Design review of the part built by this model. Coordinates are the model's own, in mm. Face numbers are marked on the shaded views. Give positions to 0.01 mm unless a question says otherwise; leave off trailing zeros. Order: outer loops, then holes, each group sorted by start corner. A loop starts at its lowest first (then second) coordinate and runs counter-clockwise, first axis right, second up. Notation, with made-up numbers: (87.25, -21) -> (98.25, -21) arc R23 cw to (98.25, -13) -> close; hole circle Ø4 at (-22, 84.5). An arc over 180 degrees is marked (long way). One line per item, written item: value.
Autodesk Inventor part; units mm, degrees
ref_plane "YZ Plane" through (0, 0, 0) normal (1, 0, 0) x (0, 1, 0)
ref_plane "XZ Plane" through (0, 0, 0) normal (0, 1, 0) x (-1, 0, 0)
ref_plane "XY Plane" through (0, 0, 0) normal (0, 0, 1) x (1, 0, 0)
sketch "Sketch1" plane through (0, 0, 0) normal (1, 0, 0) x (0, 1, 0)
  line L0 (0, 0) -> (10, 0)
  line L1 (10, 0) -> (10, -3.5)
  line L2 (10, -3.5) -> (0, -3.5)
  line L3 (0, -3.5) -> (0, 0)
  line L4 (10, -3.5) -> (0, -3.5)
  line L5 (0, -3.5) -> (0, -6)
  line L6 (0, -6) -> (10, -6)
  line L7 (10, -6) -> (10, -3.5)
  line L8 (10, -6) -> (0, -6)
  line L9 (0, -6) -> (0, -9.5)
  line L10 (0, -9.5) -> (10, -9.5)
  line L11 (10, -9.5) -> (10, -6)
  line L12 (10, -9.5) -> (0, -9.5)
  line L13 (0, -9.5) -> (0, -12)
  line L14 (0, -12) -> (10, -12)
  line L15 (10, -12) -> (10, -9.5)
  line L16 (10, -12) -> (0, -12)
  line L17 (0, -12) -> (0, -15.5)
  line L18 (0, -15.5) -> (10, -15.5)
  line L19 (10, -15.5) -> (10, -12)
  line L20 (10, -7.75) -> (5, -7.75)
  circle A0 centre (5, -7.75) radius 1.75
  line L21 (6.75, -9.5) -> (3.25, -9.5)
  line L22 (3.25, -9.5) -> (3.25, -6)
  line L23 (3.25, -6) -> (6.75, -6)
  line L24 (6.75, -6) -> (6.75, -9.5)
  line L25 (6.75, -9.5) -> (3.25, -6) construction
  line L26 (3.25, -9.5) -> (6.75, -6) construction
  dimension "d0" = 10
  dimension "d1" = 3.5
  dimension "d2" = 2.5
  dimension "d3" = 3.5
  dimension "d4" = 2.5
  dimension "d5" = 3.5
  dimension "d8" = 3.5
  dimension "d11" = 3.5
extrude "Extrusion1" add sketch "Sketch1" along normal blind 2 contours L0 L1 L2 L3 | L2 L7 L6 L5 | L6 L22 L10 L9 | L11 L20 L24 L6 | L6 A0 L22 | L10 L15 L14 L13 | L24 A0 L6 | L11 L10 L24 L20 | A0 L10 L22 | L14 L19 L18 L17 | L24 L10 A0
properties part number "yellow_plate_screw_grip_2"
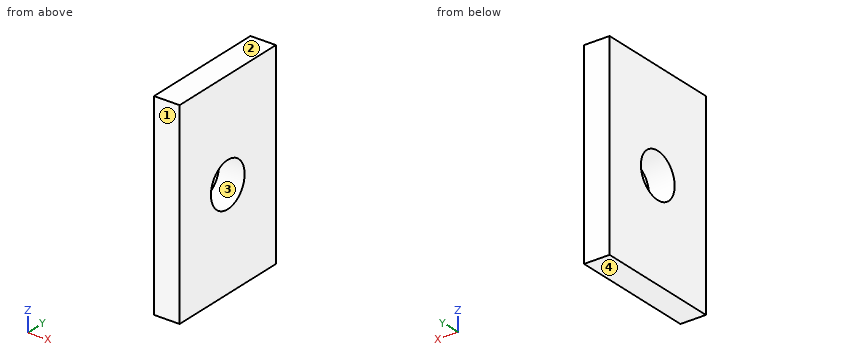
Item 1: Add section A-A on z = -7.75. Give the boundary of the cut face in (x, y).
Returned:
outline: (0, 0) -> (2, 0) -> (2, 3.25) -> (0, 3.25) -> close; (0, 6.75) -> (2, 6.75) -> (2, 10) -> (0, 10) -> close
Item 2: Add section B-B on y = 5. Give the boundary of the cut face in (x, z).
Returned:
outline: (0, -15.5) -> (2, -15.5) -> (2, -9.5) -> (0, -9.5) -> close; (0, -6) -> (2, -6) -> (2, 0) -> (0, 0) -> close
Item 3: Add section C-C on x = 0.9. Give the boundary of the cut face in (y, z).
Returned:
outline: (0, -15.5) -> (10, -15.5) -> (10, 0) -> (0, 0) -> close; hole circle Ø3.5 at (5, -7.75)
Item 4: Draft analysis for pull direction Z (two halves, no side actions). For the marked faces 1, 2, 3 and 4, state which applies: pulls with the +Z half, pulls with the -Z half, needs draft (parallel to the pull), parting line crosses it, or undercut.
Returned:
face 1: needs draft
face 2: pulls with the +Z half
face 3: undercut
face 4: pulls with the -Z half
Item 5: To check wall thickness, follow line 1 along Y through (x, z) = (0.4, -7.75); line 2 along Z through (x, y) = (0.55, 5); line 3 along Z through (x, y) = (1.25, 6.25). State the ranges of each line that lie inside material, in increasing order. Write a range as from..to.
Returned:
line 1: 0..3.25, 6.75..10
line 2: -15.5..-9.5, -6..0
line 3: -15.5..-8.97, -6.53..0
